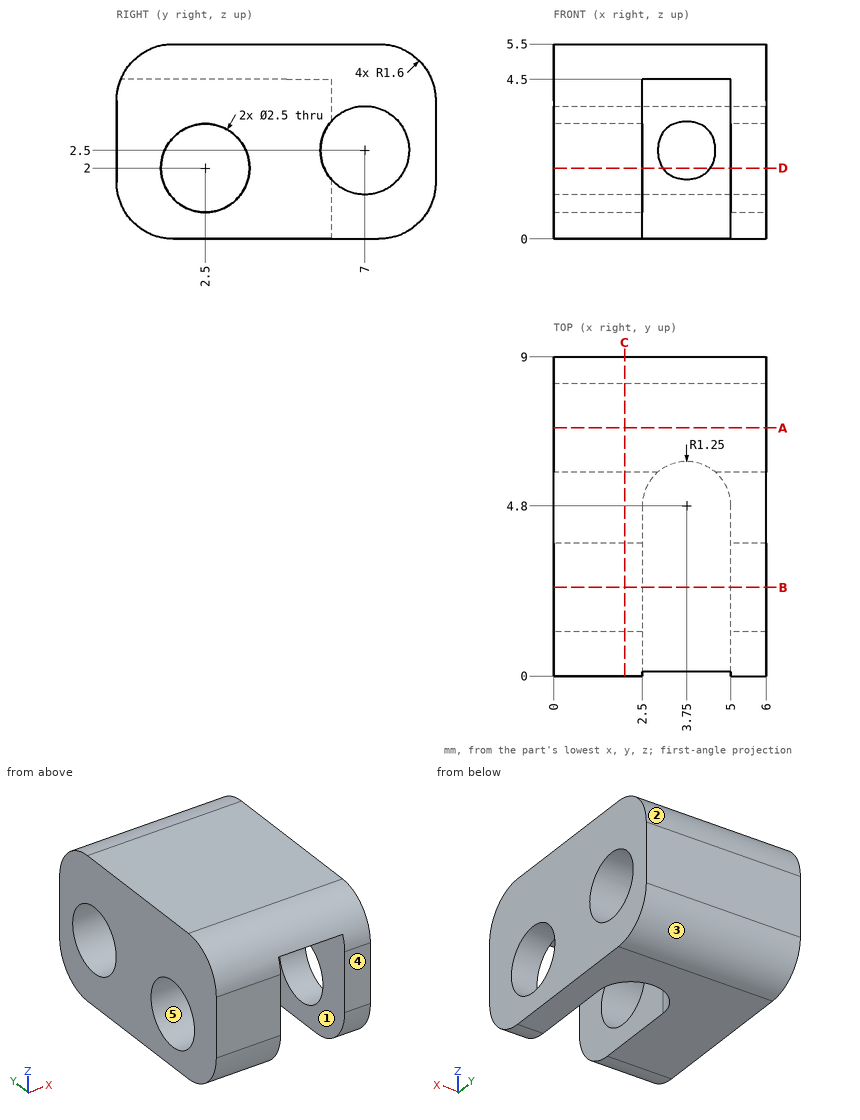
Check sheet for the drawn part. Datum: minimum x, y, z corner. Units: mm. A direction names the side the tool comes from. Give positions to 0.01 mm unless a question says otherwise; leave off trailing zeros. Order: outer loops, then holes, each group sorted by start corner. A loop starts at its lowest first (then second) coordinate and runs counter-clockwise, first axis right, second up. Notation, with made-up numbers: (48.5, -17.75) - (54.5, -17.75) arc R11 ccw to (54.5, -3.75) - close; hole circle Ø5 at (-2.5, 27.25). An arc over 180 degrees is marked (long way). Answer in a Markdown table with one row per item. Add a question column.
Q1. Cross-section at D-D, the plane z = 2. Enter the section's corners in (x, y).
Q2. Mould release check, pull along Y, two halves, no side actions. Record for the marked faces 3, 4 and 5: pulls with the +Y half, pulls with the -Y half, needs draft (parallel to the pull), parting line crosses it, or undercut.
Q3. Cross-section at B-B, the plane y = 2.5. Enter the section's corners in (x, z), then the cut area to 3 significant figures.
Q4. Material ranges on probe 1 along X at (y, z) = (3.75, 0.35); probe 2 along Z at (x, y) = (1.5, 2.5); probe 3 along Y at (x, z) = (5.7, 2), recorded low to high. Write a range as from..to.
Q5. Cross-section at C-C, the plane x = 2. Enter the section's corners in (y, z).
Q6. Cross-section at A-A, the plane y = 7. Enter the section's corners in (x, z).
Q7. Gauge pin test, flat ends, axial feed: pin 1 (1.5 mm diameter, centred on x = 3.5, z = 5, fed in from +Y); pin 2 (2 mm diameter, centred on y = 2.5, z = 2, fed in from +X); pin 3 (0.8 mm diameter, centred on x = 4, y = 4.5, fed in from -Z). Record the tip position at first contact, or that the pin passes through.
Q8. Tool access check on the marked faces 1 and 2. Record the directions out of +Z, -Z, +X, -X, +Y, -Y that give a thin tool (end or side, any length) a straight path to the whole face; none if there is none.
Check values:
| question | item | result |
|---|---|---|
| 1 | outline | (0, 0) - (2.5, 0) - (2.5, 1.25) - (0, 1.25) - close; (0, 3.75) - (2.5, 3.75) - (2.5, 4.8) arc R1.25 cw to (3.08, 5.85) - (0, 5.85) - close; (0, 8.15) - (6, 8.15) - (6, 9) - (0, 9) - close; (4.42, 5.85) arc R1.25 cw to (5, 4.8) - (5, 3.75) - (6, 3.75) - (6, 5.85) - close; (5, 0) - (6, 0) - (6, 1.25) - (5, 1.25) - close |
| 2 | face 3 | pulls with the +Y half |
| 2 | face 4 | pulls with the -Y half |
| 2 | face 5 | undercut |
| 3 | outline | (0, 0) - (2.5, 0) - (2.5, 0.75) - (0, 0.75) - close; (0, 3.25) - (2.5, 3.25) - (2.5, 4.5) - (5, 4.5) - (5, 3.25) - (6, 3.25) - (6, 5.5) - (0, 5.5) - close; (5, 0) - (6, 0) - (6, 0.75) - (5, 0.75) - close |
| 3 | area | 13.0 mm^2 |
| 4 | probe 1 | x = 0..2.5, 5..6 |
| 4 | probe 2 | z = 0..0.75, 3.25..5.5 |
| 4 | probe 3 | y = 0..1.25, 3.75..5.85, 8.15..9 |
| 5 | outline | (0, 1.6) arc R1.6 ccw to (1.6, 0) - (7.4, 0) arc R1.6 ccw to (9, 1.6) - (9, 3.9) arc R1.6 ccw to (7.4, 5.5) - (1.6, 5.5) arc R1.6 ccw to (0, 3.9) - close; hole circle Ø2.5 at (2.5, 2); hole circle Ø2.5 at (7, 2.5) |
| 6 | outline | (0, 0) - (6, 0) - (6, 1.25) - (0, 1.25) - close; (0, 3.75) - (6, 3.75) - (6, 5.5) - (0, 5.5) - close |
| 7 | pin 1 | stops at y = 8.96 |
| 7 | pin 2 | passes through |
| 7 | pin 3 | stops at z = 4.5 |
| 8 | face 1 | -Z, -Y |
| 8 | face 2 | +Z, +X, -X, +Y |
